Autodesk Inventor part; units mm, degrees
ref_plane "YZ Plane" through (0, 0, 0) normal (1, 0, 0) x (0, 1, 0)
ref_plane "XZ Plane" through (0, 0, 0) normal (0, 1, 0) x (-1, 0, 0)
ref_plane "XY Plane" through (0, 0, 0) normal (0, 0, 1) x (1, 0, 0)
sketch "Sketch1" plane through (0, 0, 0) normal (0, 0, 1) x (1, 0, 0)
  line L0 (2.3812, -1.3748) -> (0, -2.7496)
  line L1 (0, -2.7496) -> (-2.3812, -1.3748)
  line L2 (-2.3812, -1.3748) -> (-2.3813, 1.3748)
  line L3 (-2.3813, 1.3748) -> (0, 2.7496)
  line L4 (0, 2.7496) -> (2.3812, 1.3748)
  line L5 (2.3812, 1.3748) -> (2.3812, -1.3748)
  circle A0 centre (0, 0) radius 1.4986
  point P0 (2.3812, 0)
  dimension "d1" = 2.9972
extrude "Extrusion1" add sketch "Sketch1" along normal blind 25.4
fillet "Fillet1" radius 0.254 5 edges at (2.3812, 0, 0) (1.1906, -2.0622, 0) (-1.1906, -2.0622, 0) (-1.1906, 2.0622, 0) (1.1906, 2.0622, 0)
fillet "Fillet2" radius 0.254 6 edges at (2.3812, 0, 25.4) (1.1906, 2.0622, 25.4) (-1.1906, 2.0622, 25.4) (-2.3812, 0, 25.4) (-1.1906, -2.0622, 25.4) (1.1906, -2.0622, 25.4)
thread "Thread1"
properties part number "Stand-Off Posts 1inch"
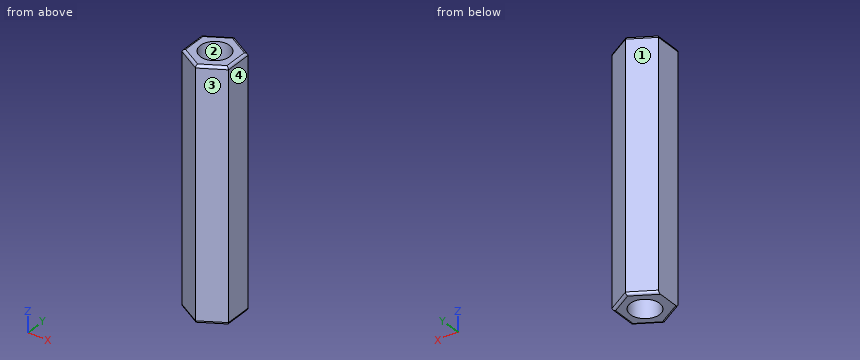
Input: part model. Units: mm. Frame: model coordinates. Face numbers are marked on the shaded views. Round coordinates to 2 decimals unless told otherwise and drop trailing zeros. Write each loop counter-clockwise with the first axis right and the second up, starting at its lowest first coordinate (ties: lowest second). Pieces come first, ordered by that corner, then holes.
1) Draft query along Y for the marked faces 1, 2, 3 and 4. Return one class per face: pulls with the +Y half, pulls with the -Y half, needs draft (parallel to the pull), parting line crosses it, or undercut.
2) Cut plane A-A (z = 3). Return the cut outline in (x, y).
3) Ray query, L1, parallel to X at y = -0.6, z = 3.75; L2, parallel to X at y = 0.8, z = 7.5; L3, parallel to Y at x = -0.05, z = 17.5. Return the intervals inside material, ascending.
Geometry says:
1. face 1: pulls with the +Y half
1. face 2: undercut
1. face 3: pulls with the -Y half
1. face 4: needs draft
2. outline: (-2.38, -1.37) - (0, -2.75) - (2.38, -1.37) - (2.38, 1.37) - (0, 2.75) - (-2.38, 1.37) - close; hole circle Ø3 at (0, 0)
3. L1: x = -2.38 to -1.37, 1.37 to 2.38
3. L2: x = -2.38 to -1.27, 1.27 to 2.38
3. L3: y = -2.72 to -1.5, 1.5 to 2.72
